Geometry: final body of the model. Coordinates: model frame, mm. A direction names the side the tool comes from. Round coordinates to 2 decimals unless told otherwise and drop trailing zeros. Write each loop counter-clockwise with the first axis right and the second up, starting at its lowest first coordinate (ties: lowest second). Pieces come first, ordered by that corner, then holes. Notation, with made-up numbers: M -6,5 L 28,5 A11 ccw 28,21 Z; hole C -13.75,-8.75 d8. An arc over 180 degrees is marked long. Put each result on its own line as item: value. Start each with the question number.
```python
from build123d import *
from OCP.BRepFilletAPI import BRepFilletAPI_MakeChamfer

# Parameters (mm, degrees)
SKETCH_1_R      = 3
EXTRUDE_1_DEPTH = 36
CHAMFER_1_SIZE  = 0.25
CHAMFER_1_SIZE2 = 0.144337567


with BuildPart() as part:
    # ｽｹｯﾁ1 → ﾎﾞｽ - 押し出し1 (new, symmetric)
    with BuildSketch(Plane.XY):
        Circle(SKETCH_1_R)
    extrude(amount=EXTRUDE_1_DEPTH, both=True)

    # 面取り1: one chamfer whose edges measure the first distance from different faces: ONE call of the kernel's chamfer builder (chamfer() names one face for all edges)
    chamfer_1_edges_1 = [part.edges().sort_by_distance(p)[0] for p in [
        (-3, 0, -36),
    ]]
    chamfer_1_side_1 = [part.faces().sort_by_distance(p)[0] for p in [
        (0, 0, -36),
    ]]
    chamfer_1_edges_2 = [part.edges().sort_by_distance(p)[0] for p in [
        (-3, 0, 36),
    ]]
    chamfer_1_side_2 = [part.faces().sort_by_distance(p)[0] for p in [
        (-3, 0, 0),
    ]]
    chamfer_1 = BRepFilletAPI_MakeChamfer(part.part.solid().wrapped)
    for e in chamfer_1_edges_1:
        chamfer_1.Add(CHAMFER_1_SIZE, CHAMFER_1_SIZE2, e.wrapped, chamfer_1_side_1[0].wrapped)  # the first distance lies on this face
    for e in chamfer_1_edges_2:
        chamfer_1.Add(CHAMFER_1_SIZE, CHAMFER_1_SIZE2, e.wrapped, chamfer_1_side_2[0].wrapped)  # the first distance lies on this face
    add(Compound.cast(chamfer_1.Shape()), mode=Mode.REPLACE)

    # ｽｹｯﾁ3 → M3x0.5 ねじ穴1 (revolve, cut)
    with BuildSketch(Plane(origin=(0, 0, 36), x_dir=(0, -1, 0), z_dir=(1, 0, 0))):
        Polygon((0, 0), (0, 13.251075774), (1.25, 12.5), (1.25, 0.275), (1.525, 0), align=None)
    m3x0_5_1 = revolve(axis=Axis((0, 0, 42.35), (0, 0, -1)), mode=Mode.SUBTRACT)

    # ﾐﾗｰ1: M3x0.5 ねじ穴1 across plane
    add(m3x0_5_1.mirror(Plane.XY), mode=Mode.SUBTRACT)


solid = part.part
```
1) Draft query along Y for faces 1 (the face through (-3, 0, 0)), 2 (the face through (1.2, -1.2, 36)), 3 (the face through (1.22, 0.27, 29.7)). Return one class per face: +Y half, -Y half, draft (parallel to the pull), parting line (faces both ways), or undercut.
2) Access query for faces 4 (the face through (1.2, -1.2, -36)), 5 (the face through (1.22, 0.27, -29.7)). Directions: +Z, -Z, +X, -X, +Y, -Y. A direction counts if a zero-diameter tool reaches every point of the face in a straight line with its end or side. Return the directions, or none.
3) Section A-A, the plane z = 4. Output: boundary loops of the cut face in (x, y), and give its area (3 significant figures).
4) First-contact query: pin 1 (3 mm diameter, centred on x = 0, y = 0, fed in from +Z) (3 decimals). Flat tip, straight axial feed; report the tip coordinate or a pass-through.
5) Ray query, probe 1 along Y at (x, z) = (0, -32.25); probe 2 along X at (y, z) = (0.9, -32); probe 3 along Y at (x, z) = (-0.55, 28). Return the intervals inside material, ascending.
Solved:
1. face 1: parting line
1. face 2: draft
1. face 3: undercut
2. face 4: -Z, +X, -X, +Y, -Y
2. face 5: -Z
3. outline: C 0,0 d6
3. area: 28.3 mm2
4. pin 1: stops at z = 35.975
5. probe 1: y = -3 to -1.25, 1.25 to 3
5. probe 2: x = -2.86 to -0.87, 0.87 to 2.86
5. probe 3: y = -2.95 to -1.12, 1.12 to 2.95
